Here's how the part is built. I have some questions about the finished solid (model axes, mm). A direction names the side the tool comes from. Coordinates: 2 decimals unless noted, no trailing zeros. Write each loop counter-clockwise with the first axis right and the second up, starting at its lowest first coordinate (ties: lowest second). Pieces come first, ordered by that corner, then holes. Notation, with made-up numbers: (65.5, 0.25) -> (71.5, 0.25) arc R36 ccw to (71.5, 36.25) -> close; hole circle Ø7 at (-11.75, -32). An arc over 180 degrees is marked (long way). Put each result on its own line as item: value. Start each with the question number.
Item 1: I want a section at D-D, the plane y = 3.45. List the corners of the cut face in (x, z) for me, then the cut area to 3 significant figures.
Item 2: For pin 1 (1 mm diameter, centred on x = -3, z = -15, fed in from -Y); pin 2 (0.9 mm diameter, centred on x = -1, y = 3, fed in from -Z); pin 3 (1.3 mm diameter, centred on y = 1.5, z = -3, fed in from +X); pin 4 (1.4 mm diameter, centred on y = 3, z = -13, fed in from -X), each with a flat end and sliding along its axis, tell me the tip position at first contact or that it passes through.
Item 3: On a 3-axis mill with a long thin cutter (end or side, diameter ignored), from which of +Z, -Z, +X, -X, +Y, -Y can I reach the whole of each face in a straight line? I mean faces 1 (the face through (0, 2, -12)), 2 (the face through (2, 3, -13)), 3 (the face through (-14, 2, 2)). Say none if no direction works.
Item 4: I want a section at B-B, the plane x = 0. List the corners of the cut face in (y, z) for me, then the cut area to 3 significant figures.
Item 5: I want a section at A-A, the plane z = 3. List the corners of the cut face in (x, y) for me, then the cut area to 3 significant figures.
Item 6: If we mould it in two halves opening along X, with no side actions, what happens to faces 4 (the face through (-15.273, 2.071, -15.949)), 5 (the face through (15.01, 2.07, -18.84)), 6 (the face through (0, 1, 12)), 7 (the face through (0, 2, 18))? For each: released by +X, released by -X, zero draft, split by the parting line, or undercut.
Item 7: I want a section at C-C, the plane y = 1. State how many separate pieces and enclosed holes the cut face has, then the cut area to 3 significant figures.
Item 8: I need wall thicknesses on line 1 (Z direction, x = 0, y = 1.75); line 2 (X direction, y = 2.9, z = 12.25); line 3 (X direction, y = 1.7, z = 14.3). Which ranges of each line are inside material? Lowest first, please. Write a range as [from, to].
from build123d import *

# Parameters (mm, degrees)
SKETCH1_R           = 1.25
SKETCH1_R_2         = 0.9
SKETCH1_W           = 12.2
SKETCH1_H           = 24
BOSS_EXTRUDE2_DEPTH = 4.2
FILLET1_R           = 3
CUT_EXTRUDE1_DEPTH  = 1.8


with BuildPart() as part:
    # Sketch1 → Boss-Extrude2 (new body)
    with BuildSketch(Plane(origin=(0, 0, 0), x_dir=(1, 0, 0), z_dir=(0, 1, 0))):
        with BuildLine():
            Line((14, -18), (14, 14))
            Line((14, 14), (16.51058682, 17.844088419))
            ThreePointArc((16.51058682, 17.844088419), (16.382617975, 20.976365727), (13.379699555, 21.876375797))
            Line((13.379699555, 21.876375797), (0, 17.690906278))
            Line((0, 17.690906278), (-13.379699555, 21.876375797))
            ThreePointArc((-13.379699555, 21.876375797), (-16.382617975, 20.976365727), (-16.51058682, 17.844088419))
            Line((-16.51058682, 17.844088419), (-14, 14))
            Line((-14, 14), (-14, -18))
            Line((-14, -18), (14, -18))
        make_face()
        with Locations(Location((-10.6, 7, 0), (0, 0, 270))):
            Circle(SKETCH1_R, mode=Mode.SUBTRACT)
        with Locations(Location((-10.6, -12.25, 0), (0, 0, 270))):
            Circle(SKETCH1_R, mode=Mode.SUBTRACT)
        with Locations(Location((-3.5, -14.3, 0), (0, 0, 270))):
            Circle(SKETCH1_R_2, mode=Mode.SUBTRACT)
        with Locations(Location((3.5, -14.3, 0), (0, 0, 270))):
            Circle(SKETCH1_R_2, mode=Mode.SUBTRACT)
        with Locations(Location((10.6, -12.25, 0), (0, 0, 270))):
            Circle(SKETCH1_R, mode=Mode.SUBTRACT)
        with Locations(Location((10.6, 7, 0), (0, 0, 270))):
            Circle(SKETCH1_R, mode=Mode.SUBTRACT)
        with Locations(Location((0, 14.3, 0), (0, 0, 270))):
            Circle(SKETCH1_R_2, mode=Mode.SUBTRACT)
        with Locations(Location((-14.25, 19.320485123, 0), (0, 0, 270))):
            Circle(SKETCH1_R_2, mode=Mode.SUBTRACT)
        with Locations(Location((14.25, 19.320485123, 0), (0, 0, 270))):
            Circle(SKETCH1_R_2, mode=Mode.SUBTRACT)
        Rectangle(SKETCH1_W, SKETCH1_H, mode=Mode.SUBTRACT)
    extrude(amount=BOSS_EXTRUDE2_DEPTH)

    # Fillet1
    fillet1_edges = [part.edges().sort_by_distance(p)[0] for p in [
        (0, 2.1, -17.690906278),
    ]]
    fillet(fillet1_edges, radius=FILLET1_R)

    # Sketch2 → Cut-Extrude1 (cut)
    with BuildSketch(Plane(origin=(0, 4.2, 0), x_dir=(1, 0, 0), z_dir=(0, 1, 0))):
        with BuildLine():
            Line((-6.1, -12), (-6.1, -14.3))
            ThreePointArc((-6.1, -14.3), (-5.338477631, -16.138477631), (-3.5, -16.9))
            Line((-3.5, -16.9), (3.5, -16.9))
            ThreePointArc((3.5, -16.9), (5.338477631, -16.138477631), (6.1, -14.3))
            Line((6.1, -14.3), (6.1, -12))
            Line((6.1, -12), (-6.1, -12))
        make_face()
        with BuildLine():
            Line((-2, 14.3), (-2, 12))
            Line((-2, 12), (2, 12))
            Line((2, 12), (2, 14.3))
            ThreePointArc((2, 14.3), (0, 16.3), (-2, 14.3))
        make_face()
    extrude(amount=-CUT_EXTRUDE1_DEPTH, mode=Mode.SUBTRACT)


solid = part.part
Calculated:
1. outline: (-16.51, -17.84) arc R2.7 ccw to (-13.38, -21.88) -> (-0.9, -17.97) arc R3 cw to (0.9, -17.97) -> (13.38, -21.88) arc R2.7 ccw to (16.51, -17.84) -> (14, -14) -> (14, 18) -> (-14, 18) -> (-14, -14) -> close; hole circle Ø1.8 at (-14.25, -19.32); hole circle Ø2.5 at (-10.6, -7); hole circle Ø2.5 at (-10.6, 12.25); hole (-6.1, -12) -> (-2, -12) -> (-2, -14.3) arc R2 ccw to (2, -14.3) -> (2, -12) -> (6.1, -12) -> (6.1, 14.3) arc R2.6 ccw to (3.5, 16.9) -> (-3.5, 16.9) arc R2.6 ccw to (-6.1, 14.3) -> close; hole circle Ø2.5 at (10.6, -7); hole circle Ø2.5 at (10.6, 12.25); hole circle Ø1.8 at (14.25, -19.32)
1. area: 702 mm2
2. pin 1: stops at y = 0
2. pin 2: stops at z = -18.14
2. pin 3: stops at x = 14
2. pin 4: stops at x = -14
3. face 1: +Y, -Y
3. face 2: +Y
3. face 3: +Z, -X, +Y, -Y
4. outline: (0, -17.83) -> (4.2, -17.83) -> (4.2, -16.3) -> (2.4, -16.3) -> (2.4, -15.2) -> (0, -15.2) -> close; (0, -13.4) -> (2.4, -13.4) -> (2.4, -12) -> (0, -12) -> close; (0, 12) -> (2.4, 12) -> (2.4, 16.9) -> (4.2, 16.9) -> (4.2, 18) -> (0, 18) -> close
4. area: 28.8 mm2
5. outline: (-14, 0) -> (-6.1, 0) -> (-6.1, 4.2) -> (-14, 4.2) -> close; (6.1, 0) -> (14, 0) -> (14, 4.2) -> (6.1, 4.2) -> close
5. area: 66.4 mm2
6. face 4: released by -X
6. face 5: undercut
6. face 6: undercut
6. face 7: zero draft
7. separate pieces: 1
7. enclosed holes: 10
7. area: 766 mm2
8. line 1: z = [-17.83, -15.2], [-13.4, -12], [12, 18]
8. line 2: x = [-14, -11.85], [-9.35, -6.1], [6.1, 9.35], [11.85, 14]
8. line 3: x = [-14, -4.4], [-2.6, 2.6], [4.4, 14]
